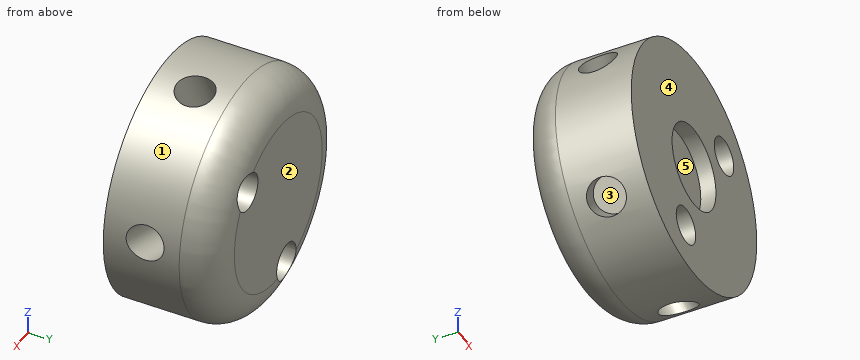
```python
from build123d import *

# Parameters (mm, degrees)
BOSS_EXTRUDE1_DEPTH        = 3
BOSS_EXTRUDE1_DEPTH_BACK   = 10
SKETCH1_R                  = 10
SKETCH4_R                  = 1.5
HOLE_DEPTH                 = 20.973741561
HOLECIR_COUNT              = 5
SKETCH6_R                  = 3.5
BEARINGHOLE_DEPTH          = 2.5
SKETCH7_R                  = 2
SHAFTHOLE_DEPTH            = 17.248076982
F_3_1_3_1_DIAMETER_HOLE1_D = 3.1
FILLET2_R                  = 3
CUT_EXTRUDE1_START         = 10
SKETCH11_R                 = 10
CUT_EXTRUDE1_DEPTH         = 10


with BuildPart() as part:
    # Sketch1 → Boss-Extrude1 (new, two sides: drawn at the far end of the back side and taken through both)
    with BuildSketch(Plane(origin=(0, 0, 0), x_dir=(1, 0, 0), z_dir=(0, 1, 0)).offset(-BOSS_EXTRUDE1_DEPTH_BACK)):
        with Locations(Location((0, 0, 0), (0, 0, 270))):
            Circle(SKETCH1_R)
    extrude(amount=BOSS_EXTRUDE1_DEPTH + BOSS_EXTRUDE1_DEPTH_BACK)

    # Sketch4 → hole (cut, through all)
    with BuildSketch(Plane(origin=(-3.352872105, -1.093066116, 1.887711608), x_dir=(-0.4486862613641547, -0.14627571033740308, -0.8816371449912632), z_dir=(0.8382180262940947, 0.2732665289126682, -0.47192790187872385))):
        with Locations(Location((0, 0, 0), (0, 0, 8.746528197))):
            Circle(SKETCH4_R)
    hole = extrude(amount=-HOLE_DEPTH, mode=Mode.SUBTRACT)

    # holecir: hole ×5 about axis
    holecir_axis = Axis((0, 0, 0), (0, 1, 0))
    for i in range(1, HOLECIR_COUNT):
        add(hole.rotate(holecir_axis, i * 360 / HOLECIR_COUNT), mode=Mode.SUBTRACT)

    # Sketch6 → bearinghole (cut)
    with BuildSketch(Plane(origin=(0, -5, 0), x_dir=(-1, 0, 0), z_dir=(0, -1, 0))):
        with Locations(Location((0, 0, 0), (0, 0, 90))):
            Circle(SKETCH6_R)
    extrude(amount=BEARINGHOLE_DEPTH, mode=Mode.SUBTRACT)

    # Sketch7 → shafthole (cut, through all)
    with BuildSketch(Plane(origin=(0, -5, 0), x_dir=(-1, 0, 0), z_dir=(0, -1, 0))):
        with Locations(Location((0, 0, 0), (0, 0, 90))):
            Circle(SKETCH7_R)
    extrude(amount=SHAFTHOLE_DEPTH, mode=Mode.SUBTRACT)

    # Ø3.1 (3.1) Diameter Hole1 (through all)
    with Locations(Plane(origin=(0, 3, 0), x_dir=(1, 0, 0), z_dir=(0, 1, 0))):
        with Locations((-1.282558474, 6.372208703), (4.783101903, -4.401356176)):
            Hole(F_3_1_3_1_DIAMETER_HOLE1_D / 2)

    # Fillet2
    # the kernel refuses this fillet: 3 mm, written as the material it takes off along each edge
    with BuildSketch(Plane(origin=(0, 3, 0), x_dir=(0, 0, 1), z_dir=(-1, 0, 0))) as fillet2_piece_1:
        with BuildLine():
            CenterArc((10 - FILLET2_R, -FILLET2_R), FILLET2_R, 0, 90)
            Line((10 - FILLET2_R, 0), (10, 0))
            Line((10, 0), (10, -FILLET2_R))
        make_face()
    revolve(axis=Axis((0, 3, 0), (0, 1, 0)), mode=Mode.SUBTRACT)
    with BuildSketch(Plane(origin=(0, -10, 0), x_dir=(0, 0, 1), z_dir=(-1, 0, 0))) as fillet2_piece_2:
        with BuildLine():
            CenterArc((10 - FILLET2_R, FILLET2_R), FILLET2_R, 270, 90)
            Line((10 - FILLET2_R, 0), (10, 0))
            Line((10, 0), (10, FILLET2_R))
        make_face()
    revolve(axis=Axis((0, -10, 0), (0, 1, 0)), mode=Mode.SUBTRACT)

    # Sketch11 → Cut-Extrude1 (cut)
    with BuildSketch(Plane(origin=(0, -6.25, 0), x_dir=(-1, 0, 0), z_dir=(0, -1, 0)).offset(CUT_EXTRUDE1_START)):
        with Locations(Location((0, 0, 0), (0, 0, 270))):
            Circle(SKETCH11_R)
    extrude(amount=-CUT_EXTRUDE1_DEPTH, mode=Mode.SUBTRACT)


solid = part.part
```
Here's how the part is built. I have some questions about the finished solid (model axes, mm). Face numbers are marked on the shaded views. A direction names the side the tool comes from. Round coordinates to 2 decimals unless told otherwise and drop trailing zeros. Answer as CSV lines item,"result".
Item 1: For pin 1 (1.5 mm diameter, centred on x = 5, y = -0.5, fed in from +Z); pin 2 (1 mm diameter, centred on x = 3.5, y = 1.5, fed in from -Z); pin 3 (4 mm diameter, centred on x = 5.5, y = -1.5, fed in from +Z), each with a flat end and sliding along its axis, tell me the tip position at first contact or that it passes through.
From the geometry:
pin 1,"z = 9.05"
pin 2,"z = -9.25"
pin 3,"z = 9.37"
Item 2: Please list where these lines run through material, in increasing order: L1, parallel to Z at x = 0, y = -5.35; L2, parallel to Z at x = -5.25, y = -2.5; L3, parallel to X at y = -1.75, z = -7.75. Write a range as [from, to].
From the geometry:
L1,"[-10, -7.24], [-5.5, -3.5], [3.5, 10]"
L2,"[-8.51, -6.87], [-3.09, 1.61], [4.56, 8.51]"
L3,"[-6.32, -1.99], [-0.57, 1.98], [4.94, 6.32]"
Item 3: Which directions (+Z, -Z, +X, -X, +Y, -Y) give clear straight access to the entire face, cutting with the end or side of a thin tool? Please do the marked faces 4 and 5.
From the geometry:
face 4,"+Z, -Z, +X, -X, -Y"
face 5,"-Y"
Item 4: Imagine slicing it at A-A on x = 5. Give the number of separate pieces and of enclosed holes in the cut face, and give its area (3 significant figures).
From the geometry:
separate pieces,"2"
enclosed holes,"1"
area,"118 mm2"
Item 5: We'd pull the mould along X, two halves only. Please class the marked faces 1, 2 and 3: +X half, -X half, draft (parallel to the pull), parting line (faces both ways), or undercut.
From the geometry:
face 1,"parting line"
face 2,"draft"
face 3,"undercut"
